from build123d import *

# Parameters (mm, degrees)
SKETCH1_R           = 17.4625
SKETCH1_R_2         = 3.175
BOSS_EXTRUDE1_DEPTH = 6.35
SKETCH3_R           = 1.651
CUT_EXTRUDE3_DEPTH  = 16.51
CHAMFER1_SIZE       = 0.762
CHAMFER2_SIZE       = 0.762


with BuildPart() as part:
    # Sketch1 → Boss-Extrude1 (new body)
    with BuildSketch(Plane.XY):
        Circle(SKETCH1_R)
        Circle(SKETCH1_R_2, mode=Mode.SUBTRACT)
    extrude(amount=BOSS_EXTRUDE1_DEPTH)

    # Sketch3 → Cut-Extrude3 (cut)
    with BuildSketch(Plane.XY.offset(6.35)):
        with Locations((0, 12.7)):
            Circle(SKETCH3_R)
    extrude(amount=-CUT_EXTRUDE3_DEPTH, mode=Mode.SUBTRACT)

    # Chamfer1
    chamfer1_edges = [part.edges().sort_by_distance(p)[0] for p in [
        (-17.4625, 0, 6.35),
    ]]
    chamfer(chamfer1_edges, length=CHAMFER1_SIZE)

    # Chamfer2
    chamfer2_edges = [part.edges().sort_by_distance(p)[0] for p in [
        (-17.4625, 0, 0),
    ]]
    chamfer(chamfer2_edges, length=CHAMFER2_SIZE)


solid = part.part
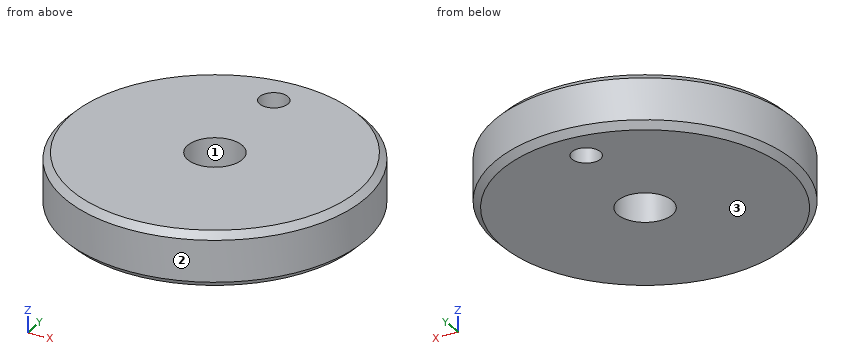
Model file for the job. Use its own axes, mm. Face numbers are marked on the shaded views. Give positions to 0.01 mm unless a question says otherwise; leave off trailing zeros. Use CSV: the item, a comma, the result in double quotes.
1. Mould opens along X. For the marked faces 1, 2 and 3 say: +X half, -X half, draft (parallel to the pull), parting line (faces both ways), or undercut.
Outcome:
face 1,"undercut"
face 2,"parting line"
face 3,"draft"
2. Drill centre lines: line 1 along Y through (x, z) = (0, 4.5) (1 decimal); line 2 along Y through (x, z) = (-0.5, 4.75); line 3 along X through (y, z) = (14, 5). Where is each one in solid material? Low to high. Write a range as from..to.
Outcome:
line 1,"-17.5..-3.2, 3.2..11, 14.4..17.5"
line 2,"-17.46..-3.14, 3.14..11.13, 14.27..17.46"
line 3,"-10.44..-1.02, 1.02..10.44"
3. Band-saw the part on A-A, the plane x = 0. Count the separate pieces of the cut face and the enclosed holes in it, then the cut area to 3 significant figures.
Outcome:
separate pieces,"3"
enclosed holes,"0"
area,"159 mm²"
4. Drop flat-ended pins along their axis: pin 1 (1 mm diameter, centred on x = -8.5, z = 2, fed in from +Y); pin 2 (4 mm diameter, centred on x = 0, y = 0, fed in from -Z); pin 3 (1 mm diameter, centred on x = 3.5, z = 5.5, fed in from -Y); pin 4 (2 mm diameter, centred on x = 3.5, z = 2.5, fed in from -Y). Give the stop position or say it passes through.
Outcome:
pin 1,"y = 15.52"
pin 2,"through"
pin 3,"y = -17.2"
pin 4,"y = -17.28"
